```python
from build123d import *

# Parameters (mm, degrees)
SKETCH_W     = 80
SKETCH_H     = 50
PAD_DEPTH    = 40
SKETCH001_R  = 10
POCKET_DEPTH = 14
FILLET_R     = 10


with BuildPart() as part:
    # Sketch → Pad (new body)
    with BuildSketch(Plane.XZ):
        Rectangle(SKETCH_W, SKETCH_H)
    extrude(amount=-PAD_DEPTH)

    # Sketch001 → Pocket (cut)
    with BuildSketch(Plane.XZ):
        with Locations((-20, 5)):
            Circle(SKETCH001_R)
    extrude(amount=-POCKET_DEPTH, mode=Mode.SUBTRACT)

    # Fillet
    fillet_edges = [part.edges().sort_by_distance(p)[0] for p in [
        (40, 20, 25),
        (40, 20, -25),
    ]]
    fillet(fillet_edges, radius=FILLET_R)


solid = part.part
```
Can you work these out from the model? Positions are in its coordinate system, mm. A direction names the side the tool comes from. Round coordinates to 2 decimals unless told otherwise and drop trailing zeros. Order: outer loops, then holes, each group sorted by start corner. A loop starts at its lowest first (then second) coordinate and runs counter-clockwise, first axis right, second up. Notation, with made-up numbers: (5, 11) -> (64, 11) arc R5 ccw to (64, 15) -> close; hole circle Ø7 at (-28.5, 21). An arc over 180 degrees is marked (long way). Return JSON: item names as keys, results as strings. Group by question number.
1. If we section it at C-C, the plane x = -20: Write out the boundary of the cut face in (y, z).
2. If we section it at D-D, the plane x = 33.5: Write out the boundary of the cut face in (y, z), then the cut area to 3 significant figures.
3. We'd pull the mould along X, two halves only. Please class faces 3 (the face through (36.99, 20.28, 22.15)), 4 (the face through (-1, 40, 0)), 5 (the face through (-10.46, 6.9, 8)): released by +X, released by -X, zero draft, split by the parting line, or undercut.
4. If we section it at B-B, the plane y = 3: Write out the boundary of the cut face in (x, z).
5. Which directions (+Z, -Z, +X, -X, +Y, -Y) give clear straight access to the entire face, cutting with the end or side of a thin tool? Please do faces 1 (the face through (-5, 20, -25)), 2 (the face through (-20, 14, 5)).
6. If we section it at A-A, the plane z = 5: Write out the boundary of the cut face in (x, y).
7. Will this pin go through, and if not, where does the flat tip stop? pin 1 (6 mm diameter, centred on x = 9, z = 6.5, fed in from -Y).
8. I need wall thicknesses on line 1 (Z direction, x = -20, y = 3); line 2 (X direction, y = 5, z = 6); line 3 (Z direction, x = -25, y = 6). Which ranges of each line are inside material? Lowest first, please. Write a range as [from, to].
Output values:
{
 "1": {"outline": "(0, -25) -> (40, -25) -> (40, 25) -> (0, 25) -> (0, 15) -> (14, 15) -> (14, -5) -> (0, -5) -> close"},
 "2": {"outline": "(0, -24.37) -> (40, -24.37) -> (40, 24.37) -> (0, 24.37) -> close", "area": "1,950 mm²"},
 "3": {"face 3": "released by +X", "face 4": "zero draft", "face 5": "undercut"},
 "4": {"outline": "(-40, -25) -> (30, -25) arc R10 ccw to (40, -15) -> (40, 15) arc R10 ccw to (30, 25) -> (-40, 25) -> close; hole circle Ø20 at (-20, 5)"},
 "5": {"face 1": "-Z, +X, -X, +Y, -Y", "face 2": "-Y"},
 "6": {"outline": "(-40, 0) -> (-30, 0) -> (-30, 14) -> (-10, 14) -> (-10, 0) -> (40, 0) -> (40, 40) -> (-40, 40) -> close"},
 "7": {"pin 1": "y = 0"},
 "8": {"line 1": "[-25, -5], [15, 25]", "line 2": "[-40, -29.95], [-10.05, 40]", "line 3": "[-25, -3.66], [13.66, 25]"}
}
